Design review of the part built by this model. Coordinates are the model's own, in mm. Face numbers are marked on the shaded views. A direction names the side the tool comes from. Give positions to 0.01 mm unless a question says otherwise; leave off trailing zeros. Order: outer loops, then holes, each group sorted by start corner. A loop starts at its lowest first (then second) coordinate and runs counter-clockwise, first axis right, second up. Notation, with made-up numbers: (-37, 54) -> (7, 54) arc R21 cw to (7, 92) -> close; hole circle Ø9 at (-3.75, 59). An arc over 180 degrees is marked (long way). One line per item, written item: value.
from build123d import *

# Parameters (mm, degrees)
SKETCH3_W                    = 15.875
SKETCH3_H                    = 15.875
CUT_EXTRUDE1_DEPTH           = 4.953
SKETCH4_W                    = 1.27
SKETCH4_H                    = 7.9375
CUT_EXTRUDE2_DEPTH           = 1.27
F_0_6_0_6_DIAMETER_HOLE1_D   = 0.6
F_2_0_2_DIAMETER_HOLE1_D     = 2
F_2_0_2_DIAMETER_HOLE1_DEPTH = 6.84
F_2_0_2_DIAMETER_HOLE1_TIP   = 0.600860619


with BuildPart() as part:
    # Sketch1 → Revolve1 (revolve)
    with BuildSketch(Plane.XY, mode=Mode.PRIVATE) as revolve1_sk:
        Polygon((-3.937, 0), (-3.937, 1.8669), (-2.921, 1.8669), (-2.921, 2.0095), (-2.43114, 2.49936), (-0.48986, 2.49936), (0, 2.0095), (0, 0), align=None)
    revolve(revolve1_sk.sketch.rotate(Axis((0, 0, 0), (-1, 0, 0)), 270), axis=Axis((0, 0, 0), (-1, 0, 0)))

    # Sketch2 → Revolve2 (revolve)
    with BuildSketch(Plane.XY, mode=Mode.PRIVATE) as revolve2_sk:
        with BuildLine():
            Line((-8.89, 0), (-8.89, 3.96875))
            Line((-8.89, 3.96875), (-8.126213706, 5.291666667))
            Line((-8.126213706, 5.291666667), (-7.177286294, 5.291666667))
            Line((-7.177286294, 5.291666667), (-6.4135, 3.96875))
            Line((-6.4135, 3.96875), (-3.937, 3.96875))
            Line((-3.937, 3.96875), (-3.937, 3.5814))
            Line((-3.937, 3.5814), (-4.2037, 3.57505))
            ThreePointArc((-4.2037, 3.57505), (-3.505192817, 2.873375), (-4.2037, 2.1717))
            Line((-4.2037, 2.1717), (-3.937, 2.1717))
            Line((-3.937, 2.1717), (-3.937, 0))
            Line((-3.937, 0), (-8.89, 0))
        make_face()
    revolve(revolve2_sk.sketch.rotate(Axis((-3.937, 0, 0), (-1, 0, 0)), 270), axis=Axis((-3.937, 0, 0), (-1, 0, 0)))

    # Sketch3 → Cut-Extrude1 (cut)
    with BuildSketch(Plane(origin=(-8.89, 0, 0), x_dir=(0, 0, -1), z_dir=(1, 0, 0))):
        Rectangle(SKETCH3_W, SKETCH3_H)
        Polygon((-4.582717762, 0), (-2.291358881, -3.96875), (2.291358881, -3.96875), (4.582717762, 0), (2.291358881, 3.96875), (-2.291358881, 3.96875), align=None, mode=Mode.SUBTRACT)
    extrude(amount=CUT_EXTRUDE1_DEPTH, mode=Mode.SUBTRACT)

    # Sketch4 → Cut-Extrude2 (cut)
    with BuildSketch(Plane(origin=(-8.89, 0, 0), x_dir=(0, 0, -1), z_dir=(1, 0, 0))):
        Rectangle(SKETCH4_W, SKETCH4_H)
    extrude(amount=CUT_EXTRUDE2_DEPTH, mode=Mode.SUBTRACT)

    # 0.6 _0.6_ Diameter Hole1 (through all)
    with Locations(Plane(origin=(0, 0, 0), x_dir=(0, 0, -1), z_dir=(1, 0, 0))):
        with Locations((0, 0)):
            Hole(F_0_6_0_6_DIAMETER_HOLE1_D / 2)

    # Sketch10 → Cut-Revolve2 (revolve, cut)
    with BuildSketch(Plane.XY, mode=Mode.PRIVATE) as cut_revolve2_sk:
        Polygon((-11.84818619, 1.090543305), (-5.946971863, 0.05), (-5.946971863, 0), (-11.84818619, 0), align=None)
    revolve(cut_revolve2_sk.sketch.rotate(Axis((0, 0, 0), (1, 0, 0)), 270), axis=Axis((0, 0, 0), (1, 0, 0)), mode=Mode.SUBTRACT)

    # 2.0 _2_ Diameter Hole1
    with Locations(Plane(origin=(0, 0, 0), x_dir=(0, 0, -1), z_dir=(1, 0, 0))):
        with Locations((0, 0)):
            Hole(F_2_0_2_DIAMETER_HOLE1_D / 2, depth=F_2_0_2_DIAMETER_HOLE1_DEPTH)
            with Locations((0, 0, -(F_2_0_2_DIAMETER_HOLE1_DEPTH + F_2_0_2_DIAMETER_HOLE1_TIP / 2))):  # 118° drill point
                Cone(0, F_2_0_2_DIAMETER_HOLE1_D / 2, F_2_0_2_DIAMETER_HOLE1_TIP, mode=Mode.SUBTRACT)


solid = part.part
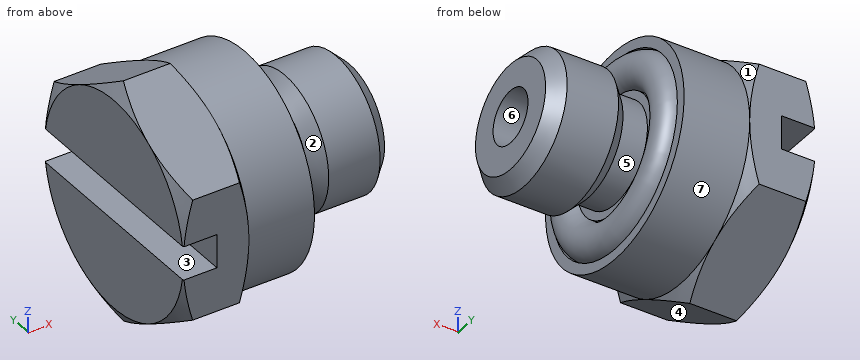
Item 1: Machinability: for the marked faces 1, 2 and 3, which of the approach directions +Z, -Z, +X, -X, +Y, -Y give a long, thin tool a straight path to every point of the face, cutting with its end or side? Answer none if there is none.
Returned:
face 1: +Z, +X, +Y
face 2: none
face 3: -X, +Y, -Y
Item 2: Add section A-A on x = -2. Give the boundary of the cut face in (y, z).
Returned:
outline: circle Ø5 at (0, 0); hole circle Ø2 at (0, 0)
Item 3: Clearance check with flat-ended pins moving along their axes: P1, Ø4, axis at x = -4, y = -1.5, coming from the +Z side; P2, Ø1, axis at x = -8, y = -1, coming from the -Z side; P3, Ø1.2, axis at y = 0, z = 0, coming from the +X side. State where each tip first meets the part, or that it passes through.
Returned:
P1: z = 3.97
P2: z = -4.29
P3: x = -7.08
Item 4: To check wall thickness, follow line 1 along Z through (x, y) = (-5.25, 0); line 2 along X through (y, z) = (3.5, -1.5). State the ranges of each line that lie inside material, in increasing order. Write a range as from..to.
Returned:
line 1: -3.97..-1, 1..3.97
line 2: -8.89..-3.94
Item 5: Draft analysis for pull direction Y (two halves, no side actions). For the marked faces 4, 5, 6 and 7, state which applies: pulls with the +Y half, pulls with the -Y half, needs draft (parallel to the pull), parting line crosses it, or undercut.
Returned:
face 4: pulls with the -Y half
face 5: undercut
face 6: undercut
face 7: parting line crosses it
